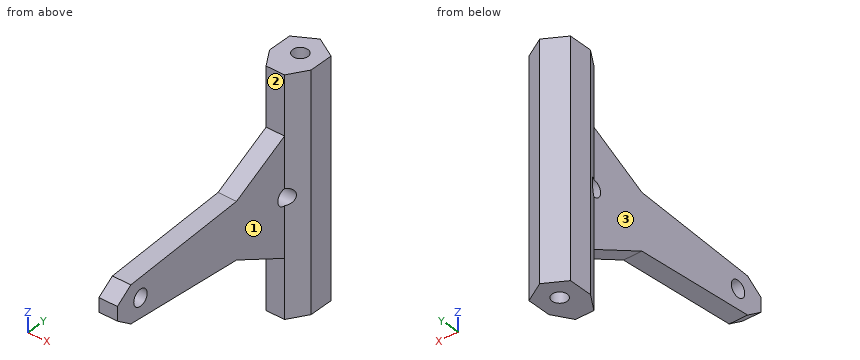
from build123d import *

# Parameters (mm, degrees)
SKETCH_1_R               = 3.25
EXTRUDE_1_DEPTH          = 100
CUT_EXTRUDE_1_DEPTH      = 143.017604543
CUT_EXTRUDE_1_DEPTH_BACK = 143.017604543
SKETCH_2_R               = 3.5


with BuildPart() as part:
    # 草圖1 → 填料-伸長1 (new body)
    with BuildSketch(Plane.XY):
        Polygon((-9, 5.196152423), (-9, -5.196152423), (-4, -13), (-4, -100), (4, -100), (4, -13), (9, -5.196152423), (9, 5.196152423), (0, 10.392304845), align=None)
        Circle(SKETCH_1_R, mode=Mode.SUBTRACT)
    extrude(amount=EXTRUDE_1_DEPTH)

    # 草圖2 → 除料-伸長1 (cut, two sides: drawn at the far end of the back side and taken through both)
    with BuildSketch(Plane.ZY.offset(4).offset(-CUT_EXTRUDE_1_DEPTH_BACK)):
        Polygon((25, -13), (0, -13), (0, -100), (47, -100), (42, -93), (38, -38), align=None)
        Polygon((58, -93), (53, -100), (100, -100), (100, -13), (75, -13), (62, -38), align=None)
        Polygon((14.096436709, -107.454844565), (0, -100), (100, -100), (75.233428016, -107.454844565), align=None)
        with BuildLine():
            Line((53.5, -13), (46.5, -13))
            ThreePointArc((46.5, -13), (50, -16.5), (53.5, -13))
        make_face()
        with BuildLine():
            ThreePointArc((53.5, -13), (50, -9.5), (46.5, -13))
            Line((46.5, -13), (53.5, -13))
        make_face()
        with Locations(Location((50, -88, 0), (0, 0, 270))):
            Circle(SKETCH_2_R)
    extrude(amount=CUT_EXTRUDE_1_DEPTH + CUT_EXTRUDE_1_DEPTH_BACK, mode=Mode.SUBTRACT)


solid = part.part
The model under review builds one solid part; all positions refer to its coordinate system, in mm. Face numbers are marked on the shaded views. A direction names the side the tool comes from. Round coordinates to 2 decimals unless told otherwise and drop trailing zeros. Loops run counter-clockwise (first coordinate to the right, second up) from the corner with the lowest first, then second, coordinate; pieces in that order, holes last. Notation, with made-up numbers: M 78.5,-27 L 92.5,-27 A20 ccw 92.5,-20 Z; hole C 66.25,-32 d1. An arc over 180 degrees is marked long. Answer as CSV lines item,"result". Start each with the question number.
Item 1: Wall thickness on line 1 (Y direction, x = 1.5, z = 50); line 2 (Y direction, x = 0.25, z = 50); line 3 (X direction, y = -22.5, z = 43.5): over which ranges is each line inside the solid? List them lowest first. Write a range as [from, to].
Item 2: Insertion check: P1, Ø9, axis at x = 0.5, z = 6.5, coming from the -Y side; P2, Ø4, axis at x = 2.5, y = -35, coming from the -Z side; P3, Ø6, axis at x = 4.5, z = 42, coming from the +Y side. Each pin has a flat end and moves straight along its axis. Give the tip position at first contact, or say it passes through.
Item 3: Consider section D-D (y = -88). Write out the cut boundary in (x, z), then the cut area to 3 significant figures.
Item 4: Consider section B-B (z = 13). Write out the cut boundary in (x, y), then the cut area to 3 significant figures.
Item 5: For the marked faces 1, 2 and 3, list the 3-axis set-ups (+Z, -Z, +X, -X, +Y, -Y) from which the entire face can be reached by the end or side of a thin tool; tool diameter is ignored.
Item 6: Consider section C-C (y = 0). Write out the cut boundary in (x, z), then the cut area to 3 significant figures.
Item 7: Consider section A-A (z = 50). Write out the cut boundary in (x, y).
Answer:
1,line 1,"y = [-100, -91.5], [-84.5, -16.5], [-9.5, -2.88], [2.88, 9.53]"
1,line 2,"y = [-100, -91.5], [-84.5, -16.5], [-9.5, -3.24], [3.24, 10.25]"
1,line 3,"x = [-4, 4]"
2,P1,"stops at y = -13"
2,P2,"stops at z = 35.4"
2,P3,"stops at y = 9.53"
3,outline,"M -4,41.64 L 4,41.64 L 4,46.5 L -4,46.5 Z; M -4,53.5 L 4,53.5 L 4,58.36 L -4,58.36 Z"
3,area,"77.8 mm^2"
4,outline,"M -9,-5.2 L -4,-13 L 4,-13 L 9,-5.2 L 9,5.2 L 0,10.39 L -9,5.2 Z; hole C 0,0 d6.5"
4,area,"302 mm^2"
5,face 1,"+Z, -Z, +X, -Y"
5,face 2,"+Z, +X, -X, -Y"
5,face 3,"+Z, -Z, -X, -Y"
6,outline,"M -9,0 L -3.25,0 L -3.25,100 L -9,100 Z; M 3.25,0 L 9,0 L 9,100 L 3.25,100 Z"
6,area,"1,150 mm^2"
7,outline,"M -9,-5.2 L -6.24,-9.5 L 6.24,-9.5 L 9,-5.2 L 9,5.2 L 0,10.39 L -9,5.2 Z; M -4,-100 L 4,-100 L 4,-91.5 L -4,-91.5 Z; M -4,-84.5 L 4,-84.5 L 4,-16.5 L -4,-16.5 Z; hole C 0,0 d6.5"
